from build123d import *

# Parameters (mm, degrees)
SKETCH1_R                   = 10.175
SKETCH1_R_2                 = 4
BOSS_EXTRUDE1_DEPTH         = 3.95
SKETCH2_R                   = 6.32
SKETCH2_R_2                 = 4
BOSS_EXTRUDE2_DEPTH         = 15.05
TAP_DRILL_FOR_M3_TAP1_D     = 2.5
TAP_DRILL_FOR_M3_TAP1_DEPTH = 3.95


with BuildPart() as part:
    # Sketch1 → Boss-Extrude1 (new body)
    with BuildSketch(Plane(origin=(0, 0, 0), x_dir=(1, 0, 0), z_dir=(0, 1, 0))):
        Circle(SKETCH1_R)
        Circle(SKETCH1_R_2, mode=Mode.SUBTRACT)
    extrude(amount=BOSS_EXTRUDE1_DEPTH)

    # Sketch2 → Boss-Extrude2 (add)
    with BuildSketch(Plane(origin=(0, 3.95, 0), x_dir=(1, 0, 0), z_dir=(0, 1, 0))):
        Circle(SKETCH2_R)
        Circle(SKETCH2_R_2, mode=Mode.SUBTRACT)
    extrude(amount=BOSS_EXTRUDE2_DEPTH)

    # Tap Drill for M3 Tap1
    with Locations(Plane(origin=(-7.144709581, 0, 4.125), x_dir=(0, 0, -1), z_dir=(0, -1, 0))):
        with Locations((0, 0), (0, 14.289419162), (12.375, 7.144709581)):
            Hole(TAP_DRILL_FOR_M3_TAP1_D / 2, depth=TAP_DRILL_FOR_M3_TAP1_DEPTH)


solid = part.part
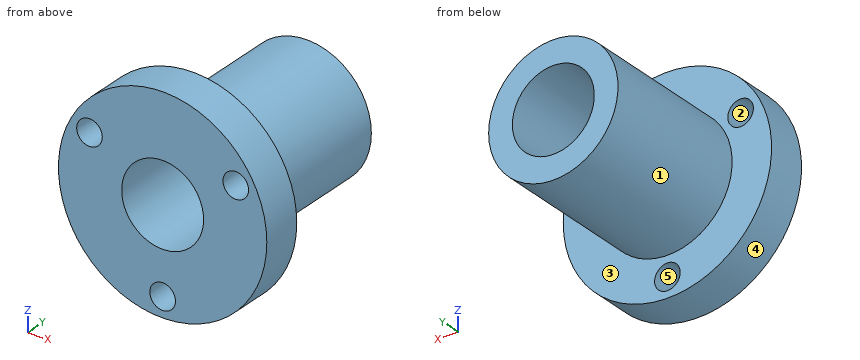
Geometry check sheet. Reference: the model listing, model coordinates, mm. Face numbers are marked on the shaded views. A direction names the side the tool comes from. Give positions to 0.01 mm unless a question says otherwise; leave off trailing zeros. Write each loop counter-clockwise with the first axis right and the second up, starting at its lowest first coordinate (ties: lowest second). Pieces come first, ordered by that corner, then holes. Notation, with made-up numbers: M 67.25,15 L 113.25,15 A25 cw 113.25,42 Z; hole C 59.25,39 d7. An arc over 180 degrees is marked long. One line per question, with ' | ' between items.
1. Cross-section at C-C (y = 11). Enter the section's corners in (x, z), plus the area to 3 significant figures.
Ans:
outline: C 0,0 d12.64; hole C 0,0 d8 | area: 75.2 mm2
2. Cross-section at D-D (z = -8.25). Enter the section's corners in (x, y).
Ans:
outline: M -5.96,0 L -1.25,0 L -1.25,3.95 L -5.96,3.95 Z; M 1.25,0 L 5.96,0 L 5.96,3.95 L 1.25,3.95 Z
3. Mould release check, pull along X, two halves, no side actions. Record for the marked faces 3, 4 and 5: released by +X, released by -X, zero draft, split by the parting line, or undercut.
Ans:
face 3: zero draft | face 4: split by the parting line | face 5: undercut
4. Cross-section at B-B (x = 0). Enter the section's corners in (y, z) (3 decimals), plus the area to 3 significant figures.
Ans:
outline: M 0,-10.175 L 3.95,-10.175 L 3.95,-9.5 L 0,-9.5 Z; M 0,-7 L 3.95,-7 L 3.95,-6.32 L 19,-6.32 L 19,-4 L 0,-4 Z; M 0,4 L 19,4 L 19,6.32 L 3.95,6.32 L 3.95,10.175 L 0,10.175 Z | area: 109 mm2
5. Set-up check for the marked faces 1 and 2: record each of +Z, -Z, +X, -X, +Y, -Y from which the full face is reachable in a straight line by a thin tool's end or side.
Ans:
face 1: +Y | face 2: +Y, -Y
6. Cross-section at A-A (z = 0). Enter the section's corners in (x, y) (3 decimals).
Ans:
outline: M -10.175,0 L -4,0 L -4,19 L -6.32,19 L -6.32,3.95 L -10.175,3.95 Z; M 4,0 L 10.175,0 L 10.175,3.95 L 6.32,3.95 L 6.32,19 L 4,19 Z
7. Gauge pin test, flat ends, axial feed: pin 1 (3 mm diameter, centred on x = -7.14, z = 4.12, fed in from +Y); pin 2 (1.5 mm diameter, centred on x = 5.5, z = -3.5, fed in from +Y); pin 3 (2 mm diameter, centred on x = 0, z = -8.25, fed in from -Y); pin 4 (1 mm diameter, centred on y = 15.5, z = 0, fed in from -X). Record the tip position at first contact, or that the pin passes through.
Ans:
pin 1: y = 3.95 | pin 2: y = 19 | pin 3: through | pin 4: x = -6.32
8. Scan lines: line 1 along X through (y, z) = (5.25, 0); line 2 along Y through (x, z) = (-3.5, 7.75). Record each from-to range of solid material in increasing order. Write a range as from..to.
Ans:
line 1: -6.32..-4, 4..6.32 | line 2: 0..3.95
